from build123d import *

# Parameters (mm, degrees)
SKETCH_1_W               = 58
SKETCH_1_H               = 58
SKETCH_1_R               = 22
SKETCH_1_R_2             = 2
EXTRUDE_1_DEPTH          = 3
SKETCH_2_R               = 22
EXTRUDE_2_DEPTH          = 20
SKETCH_4_R               = 22
SKETCH_5_R               = 22
EXTRUDE_3_DEPTH          = 45
CUT_EXTRUDE_1_DEPTH      = 5
CUT_EXTRUDE_1_DEPTH_BACK = 5
SKETCH_6_R               = 43.5
SKETCH_11_R              = 25
SKETCH_11_R_2            = 22
EXTRUDE_7_DEPTH          = 3
SKETCH_12_R              = 25
SKETCH_12_R_2            = 22
EXTRUDE_8_DEPTH          = 10
SKETCH2_R                = 11.9
SKETCH2_R_2              = 7
SKETCH2_R_3              = 1.25
EXTRUDE1_DEPTH           = 4
CUT_EXTRUDE1_DEPTH       = 51
CUT_EXTRUDE2_DEPTH       = 3
SKETCH5_R                = 2.5
CUT_EXTRUDE3_DEPTH       = 10


with BuildPart() as part:
    # 草图1 → 凸台-拉伸1 (new body)
    with BuildSketch(Plane.XY):
        with Locations((0, 29)):
            Rectangle(SKETCH_1_W, SKETCH_1_H)
        with Locations((0, 29)):
            Circle(SKETCH_1_R, mode=Mode.SUBTRACT)
        with Locations((-25, 54)):
            Circle(SKETCH_1_R_2, mode=Mode.SUBTRACT)
        with Locations((25, 54)):
            Circle(SKETCH_1_R_2, mode=Mode.SUBTRACT)
        with Locations((25, 4)):
            Circle(SKETCH_1_R_2, mode=Mode.SUBTRACT)
        with Locations((-25, 4)):
            Circle(SKETCH_1_R_2, mode=Mode.SUBTRACT)
    extrude(amount=EXTRUDE_1_DEPTH)

    # 草图2 → 凸台-拉伸2 (add)
    with BuildSketch(Plane.XY.offset(3)):
        Polygon((-25, 44), (-15, 54), (15, 54), (25, 44), (25, 14), (15, 4), (-15, 4), (-25, 14), align=None)
        with Locations((0, 29)):
            Circle(SKETCH_2_R, mode=Mode.SUBTRACT)
    extrude(amount=EXTRUDE_2_DEPTH)

    # 扫描1: sweep along a path in 草图3
    with BuildLine(Plane(origin=(0, 0, 0), x_dir=(0, 0, -1), z_dir=(1, 0, 0))) as sweep_1_path:
        ThreePointArc((-62.467090073, 56.63515398), (-47.090210327, 36.59561414), (-23, 29))
    # 草图4 → 扫描1 (sweep)
    with BuildSketch(Plane.XY.offset(23)):
        Polygon((-25, 44), (-25, 14), (-15, 4), (15, 4), (25, 14), (25, 44), (15, 54), (-15, 54), align=None)
        with Locations((0, 29)):
            Circle(SKETCH_4_R, mode=Mode.SUBTRACT)
    sweep(path=sweep_1_path.line)

    # 草图5 → 凸台-拉伸3 (add)
    with BuildSketch(Plane(origin=(0, 70.086635242, 25.509449048), x_dir=(1, 0, 0), z_dir=(0, 0.9396926207859096, 0.34202014332566555))):
        Polygon((-15, -14.329500102), (-25, -24.329500102), (-25, -54.329500102), (-15, -64.329500102), (15, -64.329500102), (25, -54.329500102), (25, -24.329500102), (15, -14.329500102), align=None)
        with Locations(Location((0, -39.329500102, 0), (0, 0, 270))):
            Circle(SKETCH_5_R, mode=Mode.SUBTRACT)
    extrude(amount=EXTRUDE_3_DEPTH)

    # 草图6 → 切除-拉伸1 (cut, two sides: drawn at the far end of the back side and taken through both)
    with BuildSketch(Plane(origin=(0, 0, 0), x_dir=(0, 0, -1), z_dir=(1, 0, 0)).offset(-CUT_EXTRUDE_1_DEPTH_BACK)):
        with Locations((-23, 71)):
            Circle(SKETCH_6_R)
    extrude(amount=CUT_EXTRUDE_1_DEPTH + CUT_EXTRUDE_1_DEPTH_BACK, mode=Mode.SUBTRACT)

    # 草图11 → 凸台-拉伸7 (add)
    with BuildSketch(Plane(origin=(0, 112.372803177, 40.900355498), x_dir=(1, 0, 0), z_dir=(0, 0.9396926207859096, 0.3420201433256655))):
        with Locations(Location((0, -39.329500102, 0), (0, 0, 270))):
            Circle(SKETCH_11_R)
        with Locations(Location((0, -39.329500102, 0), (0, 0, 103.136558787))):
            Circle(SKETCH_11_R_2, mode=Mode.SUBTRACT)
    extrude(amount=EXTRUDE_7_DEPTH)

    # 草图12 → 凸台-拉伸8 (add)
    with BuildSketch(Plane(origin=(0, 115.19188104, 41.926415928), x_dir=(1, 0, 0), z_dir=(0, 0.9396926207859096, 0.34202014332566555))):
        with Locations(Location((0, -39.329500102, 0), (0, 0, 270))):
            Circle(SKETCH_12_R)
        with Locations(Location((0, -39.329500102, 0), (0, 0, 103.136558787))):
            Circle(SKETCH_12_R_2, mode=Mode.SUBTRACT)
    extrude(amount=EXTRUDE_8_DEPTH)

    # Sketch2 → Extrude1 (add)
    # profile 1 of 2: a face of its own
    with BuildSketch(Plane(origin=(-16, 0, 0), x_dir=(0, 0, -1), z_dir=(1, 0, 0))):
        with BuildLine():
            ThreePointArc((-11.1, 71), (-31.039523471, 62.226399692), (-24.037153339, 82.854716907))
            Line((-24.037153339, 82.854716907), (-46.297321767, 80.907204522))
            Line((-46.297321767, 80.907204522), (-37.464873971, 56.640253643))
            Line((-37.464873971, 56.640253643), (-28.143847274, 52.683572923))
            Line((-28.143847274, 52.683572923), (-5.77234161, 52.683572923))
            Line((-5.77234161, 52.683572923), (-11.505482667, 74.079946637))
            ThreePointArc((-11.505482667, 74.079946637), (-11.20180615, 72.553261687), (-11.1, 71))
        make_face()
    # profile 2 of 2: a face of its own
    with BuildSketch(Plane(origin=(-16, 0, 0), x_dir=(0, 0, -1), z_dir=(1, 0, 0))):
        with Locations((-23, 71)):
            Circle(SKETCH2_R)
        with Locations((-23, 71)):
            Circle(SKETCH2_R_2, mode=Mode.SUBTRACT)
        with Locations((-14.772758664, 66.25)):
            Circle(SKETCH2_R_3, mode=Mode.SUBTRACT)
        with Locations((-31.227241336, 66.25)):
            Circle(SKETCH2_R_3, mode=Mode.SUBTRACT)
        with Locations((-23, 80.5)):
            Circle(SKETCH2_R_3, mode=Mode.SUBTRACT)
    extrude(amount=EXTRUDE1_DEPTH)

    # Sketch3 → Cut-Extrude1 (cut)
    with BuildSketch(Plane(origin=(25, 0, 0), x_dir=(0, 0, -1), z_dir=(1, 0, 0))):
        with BuildLine():
            Line((-68.96892389, 86.194013177), (-76.486464856, 83.457852031))
            ThreePointArc((-76.486464856, 83.457852031), (-78.179327787, 81.906628953), (-78.279482288, 79.612713738))
            Line((-78.279482288, 79.612713738), (-69.044938419, 54.241012977))
            ThreePointArc((-69.044938419, 54.241012977), (-51.105245381, 30.86154983), (-23, 22))
            Line((-23, 22), (-16, 22))
            ThreePointArc((-16, 22), (-13.878679656, 22.878679656), (-13, 25))
            Line((-13, 25), (-13, 33))
            ThreePointArc((-13, 33), (-13.878679656, 35.121320344), (-16, 36))
            Line((-16, 36), (-23, 36))
            ThreePointArc((-23, 36), (-43.075175272, 42.32967845), (-55.889241728, 59.029294984))
            Line((-55.889241728, 59.029294984), (-65.123785597, 84.400995745))
            ThreePointArc((-65.123785597, 84.400995745), (-66.675008674, 86.093858676), (-68.96892389, 86.194013177))
        make_face()
    extrude(amount=-CUT_EXTRUDE1_DEPTH, mode=Mode.SUBTRACT)

    # Sketch4 → Cut-Extrude2 (cut)
    with BuildSketch(Plane(origin=(0, 0, 0), x_dir=(-1, 0, 0), z_dir=(0, 0, -1))):
        Polygon((-26, 16.795799061), (-29, 19.795799061), (-29, 10.7), (-26, 13.7), align=None)
        Polygon((-26, 43.7), (-29, 46.7), (-29, 37.604200939), (-26, 40.604200939), align=None)
        Polygon((26, 40.604200939), (29, 37.604200939), (29, 46.7), (26, 43.7), align=None)
        Polygon((29, 19.795799061), (26, 16.795799061), (26, 13.7), (29, 10.7), align=None)
    extrude(amount=-CUT_EXTRUDE2_DEPTH, mode=Mode.SUBTRACT)

    # Sketch5 → Cut-Extrude3 (cut)
    with BuildSketch(Plane(origin=(0, -22.001984845, 60.449956545), x_dir=(1, 0, 0), z_dir=(0, -0.3420201433256656, 0.9396926207859096))):
        with Locations(Location((0, 114.584639372, 0), (0, 0, 270))):
            Circle(SKETCH5_R)
    extrude(amount=-CUT_EXTRUDE3_DEPTH, mode=Mode.SUBTRACT)


solid = part.part
Check sheet for the modelled part. Datum: model origin and axes. Units: mm. A direction names the side the tool comes from. Give positions to 0.01 mm unless a question says otherwise; leave off trailing zeros. Answer as a JSON object with one key per item and string values. Group by question number.
Q1. Cross-section at A-A on y = 71. Give the number of separate pieces and of enclosed holes in the cut face, then the cut area to 3 significant figures.
Q2. Release check for a two-part mould opening along Y. For faces 4 (the flat face through (29, 29, 1)), 5 (the flat face through (-17, 58, 1)), 6 (the cylindrical face through (22.957, 81.936, 78.165)) record: released by +Y, released by -Y, zero draft, split by the parting line, or undercut.
Q3. Go/stop test with flat-tipped pins: P1, Ø1.5, axis at y = 42.5, z = 2, coming from the +X side; P2, Ø1.7, axis at x = 23, y = 28.5, coming from the +Z side; P3, Ø22.5, axis at y = 71, z = 23, coming from the -X side; P4, Ø3.5, axis at x = 25, y = 4, coming from the -Z side. Record where each tip stops, or that it passes through.
Q4. Access from +Z, -Z, +X, -X, +Y, -Y to the whole of each face (thin tool, end or side, straight path). Record for faces 1 (the cylindrical face through (-22.9, 22.86, 13.9)), 2 (the flat face through (-25, 57, 51)), 3 (the cylindrical face through (-0.07, 101.446, 54.069)).
Q5. Material ranges on line 1 along Y through (x, z) = (-25, 1); line 2 along Z through (x, y) = (-13.3, 80.5); line 3 along Y through (x, z) = (0, 8.75), recorded low to high. Write a range as [from, to].
Evaluation:
{
 "1": {"separate pieces": "4", "enclosed holes": "0", "area": "761 mm2"},
 "2": {"face 4": "zero draft", "face 5": "released by +Y", "face 6": "undercut"},
 "3": {"P1": "stops at x = 26", "P2": "stops at z = 65.41", "P3": "stops at x = -16", "P4": "passes through"},
 "4": {"face 1": "+X, -X", "face 2": "+Z, -X, +Y, -Y", "face 3": "-Z"},
 "5": {"line 1": "y = [0, 2], [6, 52], [56, 58]", "line 2": "z = [15.83, 21.75], [24.25, 52.5], [89.8, 97.76]", "line 3": "y = [4, 7]"}
}
